from build123d import *

# Parameters (mm, degrees)
SKETCH1_W                = 54
SKETCH1_H                = 37.4
BOSS_EXTRUDE1_DEPTH      = 2
CUT_EXTRUDE1_DEPTH       = 54.160020758
SKETCH4_R                = 3
SKETCH4_R_2              = 1.5
BOSS_EXTRUDE2_DEPTH      = 4
BOSS_EXTRUDE3_REACH      = 75.013
BOSS_EXTRUDE3_END_RADIUS = 3
SKETCH6_W                = 4
SKETCH6_H                = 6
LOFT1_START              = -48.911518112
LOFT1_DEPTH              = 4
SKETCH8_2_W              = 4
SKETCH8_2_H              = 6
BOSS_EXTRUDE4_DEPTH      = 2
FILLET5_R                = 2
FILLET1_R                = 4
FILLET2_R                = 4
FILLET3_R                = 4
INTERSECT1_START         = -9.028476462
INTERSECT1_OUTLINE_W     = 54
INTERSECT1_OUTLINE_H     = 2
INTERSECT1_DEPTH         = 18.7
INTERSECT2_START         = -17.911518112
INTERSECT2_OUTLINE_W     = 18.7
INTERSECT2_OUTLINE_H     = 2
INTERSECT2_DEPTH         = 27


# Read off the part's stored shape, not the designer's step: Loft1, Intersect1, Intersect2
with BuildPart() as part:
    # Sketch1 → Boss-Extrude1 (new body)
    with BuildSketch(Plane.XY):
        with Locations((-17.911518112, 9.671523538)):
            Rectangle(SKETCH1_W, SKETCH1_H)
    extrude(amount=BOSS_EXTRUDE1_DEPTH)

    # Sketch2 → Cut-Extrude1 (cut, through all)
    with BuildSketch(Plane.XY.offset(2)):
        Polygon((-22.764922959, 24.371523538), (-29.981326879, 19.759300163), (-37.197730799, 24.371523538), align=None)
        Polygon((-33.695114192, 17.385705663), (-40.911518112, 12.773482289), (-40.911518112, 21.997929038), align=None)
        Polygon((-29.981326879, 15.012111163), (-37.408901505, 10.264922163), (-29.052880051, 4.924334538), (-21.625305425, 9.671523538), align=None)
        Polygon((-18.83996494, 22.132894663), (-26.267539566, 17.385705663), (-17.911518112, 12.045118038), (-10.483943486, 16.792307038), align=None)
        Polygon((1.374694575, 24.371523538), (-14.915006921, 24.371523538), (-6.770156173, 19.165901538), align=None)
        Polygon((-3.05636886, 16.792307038), (5.088481888, 11.586685039), (5.088481888, 21.997929038), align=None)
        Polygon((-6.770156173, 14.418712538), (-14.197730799, 9.671523538), (-5.841709344, 4.330935913), (1.585865282, 9.078124913), align=None)
        Polygon((-17.911518112, 7.297929038), (-25.339092738, 2.550740038), (-16.983071283, -2.789847587), (-9.555496657, 1.957341413), align=None)
        Polygon((-29.052880051, 0.177145538), (-20.908029303, -5.028476462), (-37.197730799, -5.028476462), align=None)
        Polygon((-40.911518112, 7.756362038), (-32.766667364, 2.550740038), (-40.911518112, -2.654881962), align=None)
        Polygon((-13.058113264, -5.028476462), (-5.841709344, -0.416253087), (1.374694575, -5.028476462), align=None)
        Polygon((-2.127922031, 1.957341413), (5.088481888, 6.569564788), (5.088481888, -2.654881962), align=None)
    extrude(amount=-CUT_EXTRUDE1_DEPTH, mode=Mode.SUBTRACT)



with BuildPart() as body_2:
    # Sketch4 → Boss-Extrude2 (new body)
    with BuildSketch(Plane.XY.offset(25)):
        with Locations((-54.911518112, 36.671523538)):
            Circle(SKETCH4_R)
        with Locations((-54.911518112, 36.671523538)):
            Circle(SKETCH4_R_2, mode=Mode.SUBTRACT)
    extrude(amount=BOSS_EXTRUDE2_DEPTH)

    # Boss-Extrude3: up to this cylinder (the profile starts outside it)
    boss_extrude3_end = Plane(origin=(-54.911518112, 36.671523538, 27), z_dir=(0, 0, -1)) * Cylinder(BOSS_EXTRUDE3_END_RADIUS, 157.026, mode=Mode.PRIVATE)
    # Sketch6 → Boss-Extrude3 (add, up to the surface)
    with BuildSketch(Plane.ZY.offset(44.911518112), mode=Mode.PRIVATE) as boss_extrude3_sk1:
        with Locations((27, 36.671523538)):
            Rectangle(SKETCH6_W, SKETCH6_H)
    boss_extrude3_tool1 = extrude(boss_extrude3_sk1.sketch, amount=BOSS_EXTRUDE3_REACH, mode=Mode.PRIVATE) - boss_extrude3_end
    add(boss_extrude3_tool1.solids().sort_by_distance((-44.911518, 36.671524, 27))[0])

    # Loft1 outline → Loft1 (add)
    with BuildSketch(Plane.YZ.offset(LOFT1_START)):
        Polygon((22.371523538, 2), (28.371523538, 2), (39.671523538, 25), (33.671523538, 25), align=None)
    extrude(amount=LOFT1_DEPTH)


with BuildPart() as part_1:
    add(part.part)

    add(body_2.part)  # Boss-Extrude4 merges body 2
    # Sketch8<2> → Boss-Extrude4 (add)
    with BuildSketch(Plane.XY.offset(2)):
        with Locations((-46.911518112, 25.371523538)):
            Rectangle(SKETCH8_2_W, SKETCH8_2_H)
    extrude(amount=-BOSS_EXTRUDE4_DEPTH)

    # Fillet5
    fillet5_edges = [part_1.edges().sort_by_distance(p)[0] for p in [
        (-48.911518112, 36.671523538, 25),
    ]]
    fillet(fillet5_edges, radius=FILLET5_R)

    # Fillet1
    # the kernel refuses this fillet: 4 mm, written as the material it adds along each edge
    with BuildSketch(Plane(origin=(-44.911518112, 22.371523538, 2), x_dir=(-1, 0, 0), z_dir=(0, 0, -1))) as fillet1_piece_1:
        with BuildLine():
            CenterArc((FILLET1_R, -FILLET1_R), FILLET1_R, 90, 90)
            Line((0, -FILLET1_R), (0, 0))
            Line((0, 0), (FILLET1_R, 0))
        make_face()
    extrude(amount=2)

    # Fillet2
    fillet2_edges = [part_1.edges().sort_by_distance(p)[0] for p in [
        (-44.911518112, 25.371523538, 2),
    ]]
    fillet(fillet2_edges, radius=FILLET2_R)

    # Fillet3
    # the kernel refuses this fillet: 4 mm, written as the material it adds along each edge
    with BuildSketch(Plane(origin=(-40.911518112, 22.371523538, 2), x_dir=(-1.1887379968908428e-11, -1.0, 0), z_dir=(-1.0, 1.188737996890843e-11, 0))) as fillet3_piece_1_section:
        with BuildLine():
            CenterArc((FILLET3_R * 0.622867973762, FILLET3_R), FILLET3_R, 206.165087136, 63.834912864)
            Line((-FILLET3_R * 0.274659258448, FILLET3_R * 0.559040968523), (0, 0))
            Line((0, 0), (FILLET3_R * 0.622867973762, 0))
        make_face()
    fillet3_piece_1 = extrude(amount=8, mode=Mode.PRIVATE)
    fillet3_piece_1 = fillet3_piece_1 - Plane(origin=(-48.911518112, 18.371523538, 2.009489355), x_dir=(-1, 0, 0), z_dir=(0, 0, 1)) * Cylinder(4, 26, mode=Mode.PRIVATE)
    fillet3_piece_1 = fillet3_piece_1 - Plane(origin=(-40.911518112, 22.302452917, 6), x_dir=(0, 0, -1), z_dir=(0, 1, 0)) * Cylinder(4, 26, mode=Mode.PRIVATE)
    add(fillet3_piece_1)

    # Intersect1 outline → Intersect1 (cut)
    with BuildSketch(Plane(origin=(0, 0, 0), x_dir=(1, 0, 0), z_dir=(0, 1, 0)).offset(INTERSECT1_START)):
        with Locations((-17.911518112, -1)):
            Rectangle(INTERSECT1_OUTLINE_W, INTERSECT1_OUTLINE_H)
    extrude(amount=INTERSECT1_DEPTH, mode=Mode.SUBTRACT)

    # Intersect2 outline → Intersect2 (cut)
    with BuildSketch(Plane.YZ.offset(INTERSECT2_START)):
        with Locations((19.021523538, 1)):
            Rectangle(INTERSECT2_OUTLINE_W, INTERSECT2_OUTLINE_H)
    extrude(amount=INTERSECT2_DEPTH, mode=Mode.SUBTRACT)

    # Mirror3: part across plane


with BuildPart() as part_2:
    add(part_1.part)
    add(part_1.part.mirror(Plane.ZY.offset(17.911518112)))

    # Mirror4: part across plane


with BuildPart() as part_3:
    add(part_2.part)
    add(part_2.part.mirror(Plane.ZX.offset(9.671523538)))


solid = part_3.part
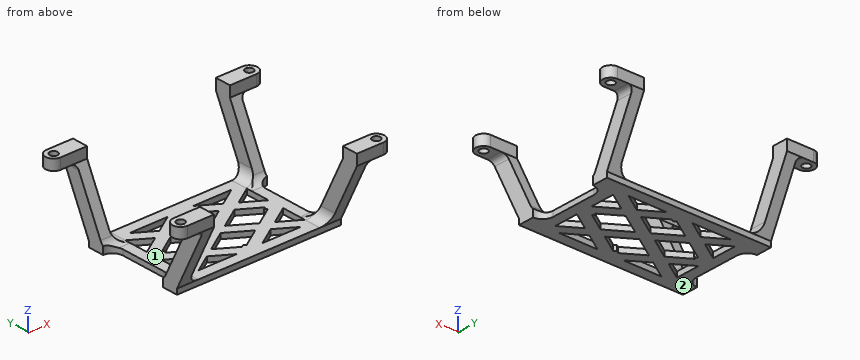
Verification items for the finished model (mm, model axes). Face numbers are marked on the shaded views. Coordinates: 2 decimals unless noted, no trailing zeros. Order: outer loops, then holes, each group sorted by start corner. A loop starts at its lowest first (then second) coordinate and runs counter-clockwise, first axis right, second up.
1. Go/stop test with flat-tipped pins: pin 1 Ø12 at (x, z) = (-30.5, 9.5) entering from -Y; pin 2 Ø4 at (x, y) = (19.09, 36.67) entering from -Z; pin 3 Ø1 at (x, z) = (-8.5, 1) entering from -Y; pin 4 Ø1.5 at (x, y) = (-4.5, 1.5) entering from -Z. Record where each tip stops, or that it passes through.
Results found:
pin 1: passes through
pin 2: stops at z = 25
pin 3: stops at y = -9.03
pin 4: stops at z = 0
2. Scan lines: line 1 (X direction, y = -7.5, z = 11); line 2 (Y direction, x = 18, z = 25.5); line 3 (Y direction, x = -47.5, z = 24.75). Record each from-to range of solid material in increasing order.
Results found:
line 1: x = -48.91 to -44.91, 9.09 to 13.09
line 2: y = -20.33 to -18.36, -16.3 to -14.33, 33.67 to 35.64, 37.7 to 39.67
line 3: y = -20.21 to -14.21, 33.55 to 39.55
3. Sectioned sample at D-D, the plane x = -12. Record the cut outline in (y, z).
Results found:
outline: (-9.03, 0) - (-5.03, 0) - (-5.03, 2) - (-9.03, 2) - close; (-4.35, 0) - (0.39, 0) - (0.39, 2) - (-4.35, 2) - close; (3.52, 0) - (8.27, 0) - (8.27, 2) - (3.52, 2) - close; (11.08, 0) - (15.82, 0) - (15.82, 2) - (11.08, 2) - close; (18.95, 0) - (23.7, 0) - (23.7, 2) - (18.95, 2) - close; (24.37, 0) - (28.37, 0) - (28.37, 2) - (24.37, 2) - close
4. Sectioned sample at B-B, the plane z = 26.25. Record the cut outline in (x, y), and give its area (3 significant figures).
Results found:
outline: (-54.91, -20.33) - (-44.91, -20.33) - (-44.91, -14.33) - (-54.91, -14.33) arc R3 ccw to start; (-54.91, 33.67) - (-44.91, 33.67) - (-44.91, 39.67) - (-54.91, 39.67) arc R3 ccw to start; (9.09, -20.33) - (19.09, -20.33) arc R3 ccw to (19.09, -14.33) - (9.09, -14.33) - close; (9.09, 33.67) - (19.09, 33.67) arc R3 ccw to (19.09, 39.67) - (9.09, 39.67) - close; hole circle Ø3 at (-54.91, -17.33); hole circle Ø3 at (-54.91, 36.67); hole circle Ø3 at (19.09, -17.33); hole circle Ø3 at (19.09, 36.67)
area: 268 mm2
5. Sectioned sample at C-C, the plane y = -12. Record the cut outline in (x, z), and give its area (3 significant figures).
Results found:
outline: (-48.91, 8.05) - (-44.91, 8.05) - (-44.91, 20.26) - (-48.91, 20.26) - close; (9.09, 8.05) - (13.09, 8.05) - (13.09, 20.26) - (9.09, 20.26) - close
area: 97.7 mm2
6. Sectioned sample at A-A, the plane x = -29. Record the cut outline in (y, z), and give its area (3 significant figures).
Results found:
outline: (-9.03, 0) - (-5.03, 0) - (-5.03, 2) - (-9.03, 2) - close; (-1.04, 0) - (4.96, 0) - (4.96, 2) - (-1.04, 2) - close; (14.38, 0) - (20.39, 0) - (20.39, 2) - (14.38, 2) - close; (24.37, 0) - (28.37, 0) - (28.37, 2) - (24.37, 2) - close
area: 40.0 mm2
7. Release check for a two-part mould opening along Y. For the marked faces 1 and 2 record: +Y half, -Y half, draft (parallel to the pull), parting line (faces both ways), or undercut.
Results found:
face 1: undercut
face 2: draft
